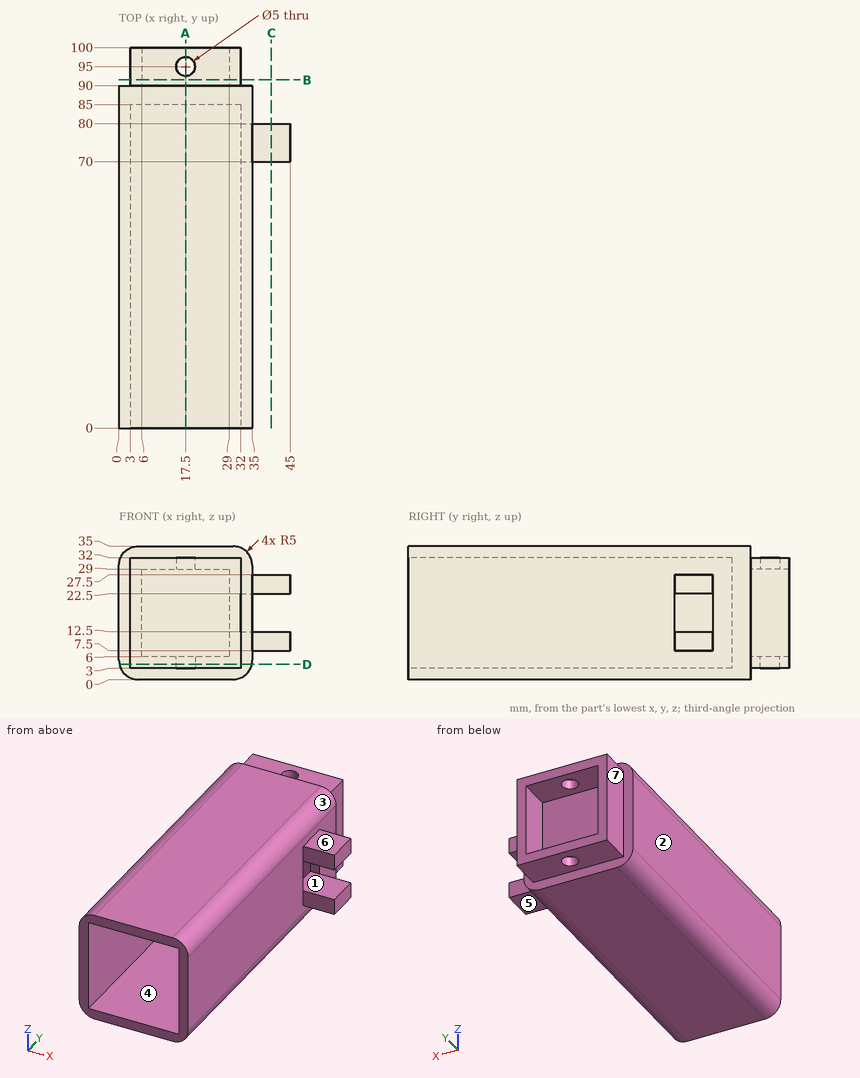
Source: three-view drawing plus pictorial views. Frame: mm from the lowest corner of the part. A direction names the side the tool comes from. Coordinates: 2 decimals unless noted, no trailing zeros. Order: outer loops, then holes, each group sorted by start corner. A loop starts at its lowest first (then second) coordinate and runs counter-clockwise, first axis right, second up.
1) Section A-A (x = 17.5). Return loops of the section in (y, z).
Result sheet:
outline: (0, 0) - (90, 0) - (90, 3) - (92.5, 3) - (92.5, 6) - (90, 6) - (90, 29) - (92.5, 29) - (92.5, 32) - (90, 32) - (90, 35) - (0, 35) - (0, 32) - (85, 32) - (85, 3) - (0, 3) - close; (97.5, 3) - (100, 3) - (100, 6) - (97.5, 6) - close; (97.5, 29) - (100, 29) - (100, 32) - (97.5, 32) - close
2) Section B-B (y = 91.5). Return loops of the section in (x, z), then the cut area to 3 significant figures.
Result sheet:
outline: (3, 3) - (32, 3) - (32, 32) - (3, 32) - close; hole (6, 6) - (29, 6) - (29, 29) - (6, 29) - close
area: 312 mm2
3) Section C-C (x = 40). Return loops of the section in (y, z), then the cut area to 3 significant figures.
Result sheet:
outline: (70, 7.5) - (80, 7.5) - (80, 12.5) - (70, 12.5) - close; (70, 22.5) - (80, 22.5) - (80, 27.5) - (70, 27.5) - close
area: 100 mm2
4) Ray query, probe 1 along Y at (x, z) = (17.5, 30.85); probe 2 along X at (y, z) = (95, 30.9); probe 3 along Z at (x, y) = (9, 83.5). Return the intervals inside material, ascending.
Result sheet:
probe 1: y = 85 to 92.5, 97.5 to 100
probe 2: x = 3 to 15, 20 to 32
probe 3: z = 0 to 3, 32 to 35
5) First-contact query: P1, Ø3, axis at x = 24, y = 94, coming from the -Z side; P2, Ø4, axis at y = 14.5, z = 14.5, coming from the +X side; P3, Ø6.5, axis at x = 17.5, y = 95, coming from the +Z side. Flat tips, straight axial feed; report the tip coordinate or a pass-through.
Result sheet:
P1: stops at z = 3
P2: stops at x = 35
P3: stops at z = 32
6) Draft query along Z for the marked faces 1, 2 and 3. Return one class per face: released by +Z, released by -Z, zero draft, split by the parting line, or undercut.
Result sheet:
face 1: undercut
face 2: zero draft
face 3: released by +Z
7) Set-up query: the marked faces 4, 5, 6 and 7. Return all of +Z, -Z, +X, -X, +Y, -Y with unobstructed straight access to the full face (end or side cutting, diameter ignored); none if empty.
Result sheet:
face 4: -Y
face 5: -Z, +X, +Y, -Y
face 6: +Z, +X, +Y, -Y
face 7: +Z, -Z, -X, +Y
8) Section D-D (z = 4). Return loops of the section in (x, y).
Result sheet:
outline: (0.1, 0) - (3, 0) - (3, 85) - (32, 85) - (32, 0) - (34.9, 0) - (34.9, 90) - (32, 90) - (32, 100) - (3, 100) - (3, 90) - (0.1, 90) - close; hole circle Ø5 at (17.5, 95)
